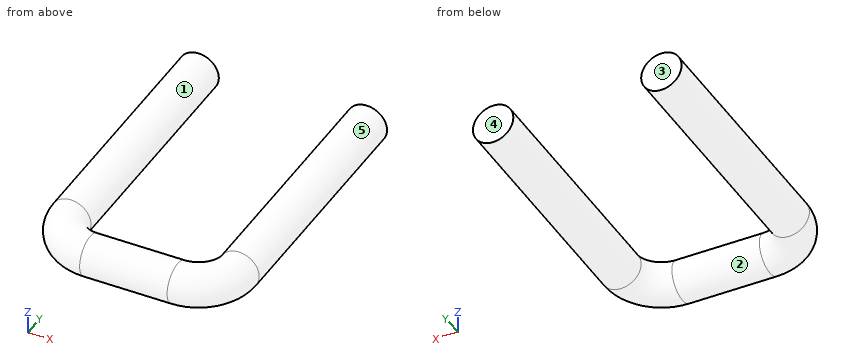
Autodesk Inventor part; units mm, degrees
ref_plane "YZ Plane" through (0, 0, 0) normal (1, 0, 0) x (0, 1, 0)
ref_plane "XZ Plane" through (0, 0, 0) normal (0, 1, 0) x (-1, 0, 0)
ref_plane "XY Plane" through (0, 0, 0) normal (0, 0, 1) x (1, 0, 0)
sketch "Sketch1" plane through (0, 0, 0) normal (1, 0, 0) x (0, 1, 0)
  circle A0 centre (0, 0) radius 6
  dimension "d0" = 12
sketch "Sketch2" plane through (0, 0, 0) normal (0, 0, 1) x (1, 0, 0)
  line L0 (0, 0) -> (13, 0)
  line L1 (25, 12) -> (25, 85)
  line L2 (0, 0) -> (0, 120)
  line L3 (0, 0) -> (-13, 0)
  line L4 (-25, 12) -> (-25, 85)
  arc A0 (-25, 12) -> (-13, 0) centre (-13, 12) ccw
  arc A1 (13, 0) -> (25, 12) centre (13, 12) ccw
  point P0 (25, 0)
  point P1 (-25, 0)
  dimension "d1" = 25
  dimension "d2" = 85
  dimension "d3" = 12
sweep "Sweep1" add profiles "Sketch1" path "Sketch2" path curves L1 A1 L0 L3 A0 L4
thread "Thread1"
thread "Thread2"
properties part number "Suspension_Clamp_U-Bolt"
Geometry: final body of the model. Coordinates: model frame, mm. Face numbers are marked on the shaded views. A direction names the side the tool comes from. Round coordinates to 2 decimals unless told otherwise and drop trailing zeros. Loops run counter-clockwise (first coordinate to the right, second up) from the corner with the lowest first, then second, coordinate; pieces in that order, holes last. Notation, with made-up numbers: (25.5, -16.5) -> (45.5, -16.5) arc R16 ccw to (45.5, 0.5) -> close; hole circle Ø5 at (60.5, 11). An arc over 180 degrees is marked (long way). Use one line per item in the form item = value.
Item 1: Contact query for flat-ended pins moving along their axis: pin 1 Ø5 at (x, z) = (-2.5, -1) entering from -Y; pin 2 Ø3 at (x, z) = (-19, 3.5) entering from -Y; pin 3 Ø6 at (x, y) = (16.5, 33) entering from -Z; pin 4 Ø12 at (x, y) = (-11, 41.5) entering from -Z. Output: stop coordinate, or through.
Evaluation:
pin_1 = -6
pin_2 = -4.78
pin_3 = -2.4
pin_4 = through
Item 2: Cut plane B-B on y = 19. Output: boundary loops of the cut face in (x, z), then the cut area to 3 significant figures.
Evaluation:
outline = circle Ø12 at (-25, 0); circle Ø12 at (25, 0)
area = 226 mm2
Item 3: Cut plane A-A on z = 0. Output: boundary loops of the cut face in (x, y), then the cut area to 3 significant figures.
Evaluation:
outline = (-31, 12) arc R18 ccw to (-13, -6) -> (13, -6) arc R18 ccw to (31, 12) -> (31, 85) -> (19, 85) -> (19, 12) arc R6 cw to (13, 6) -> (-13, 6) arc R6 cw to (-19, 12) -> (-19, 85) -> (-31, 85) -> close
area = 2,520 mm2
Item 4: Material intervals for probe 1 along X at (y, z) = (72, -3.75); probe 2 along X at (y, z) = (16, 0.75); probe 3 along Z at (x, y) = (-23.5, 67), sorted ascending.
Evaluation:
probe_1 = -29.68 to -20.32, 20.32 to 29.68
probe_2 = -30.95 to -19.05, 19.05 to 30.95
probe_3 = -5.81 to 5.81
Item 5: Draft query along X for the marked faces 4 and 5. Return one class per face: released by +X, released by -X, zero draft, split by the parting line, or undercut.
Evaluation:
face_4 = zero draft
face_5 = undercut
Item 6: Access query for the marked faces 1, 2 and 3. Directions: +Z, -Z, +X, -X, +Y, -Y. A direction counts if a zero-diameter tool reaches every point of the face in a straight line with its end or side. Return the directions, or none.
Evaluation:
face_1 = +Y
face_2 = none
face_3 = +Z, -Z, +X, -X, +Y
